Here's the drawing with two shaded views (mm, measured from the low corner). I have some questions. Round coordinates to 2 decimals unless told otherwise and drop trailing zeros. Loops run counter-clockwise (first coordinate to the right, second up) from the corner with the lowest first, then second, coordinate; pieces in that order, holes last.
(1) I want a section at B-B on y = 9. Write out the boundary of the cut face in (x, z).
(2) Will these pins go through, and if not, where does the flat tip stop? pin 1 Ø1.8 at (x, z) = (25, 7.5) entering from -Y; pin 2 Ø1.6 at (x, z) = (31.5, 0.5) entering from -Y; pin 3 Ø10 at (x, y) = (23.5, 45) entering from +Z; pin 4 Ø1.2 at (y, z) = (59, 4) entering from +X.
(3) I want a section at C-C on z = 7.5. Write out the boundary of the cut face in (x, y), plus the area to 3 significant figures.
(4) I want a section at A-A on x = 10. Write out the boundary of the cut face in (y, z).
(5) I want a section at D-D on x = 29. Write out the boundary of the cut face in (y, z).
(6) If I drill on line 1 along X through (y, z) = (51, 0.9); line 2 along Y through (x, z) = (4.5, 0.85); line 3 along Y through (x, z) = (15, 1), over which ranges is the centre line in solid material (lowest first)?
(7) Thinking about a two-plate mould opening in Y: for the marked faces 1, 2, 3 and 4, which applies, released by +Y, released by -Y, zero draft, split by the parting line, or undercut?
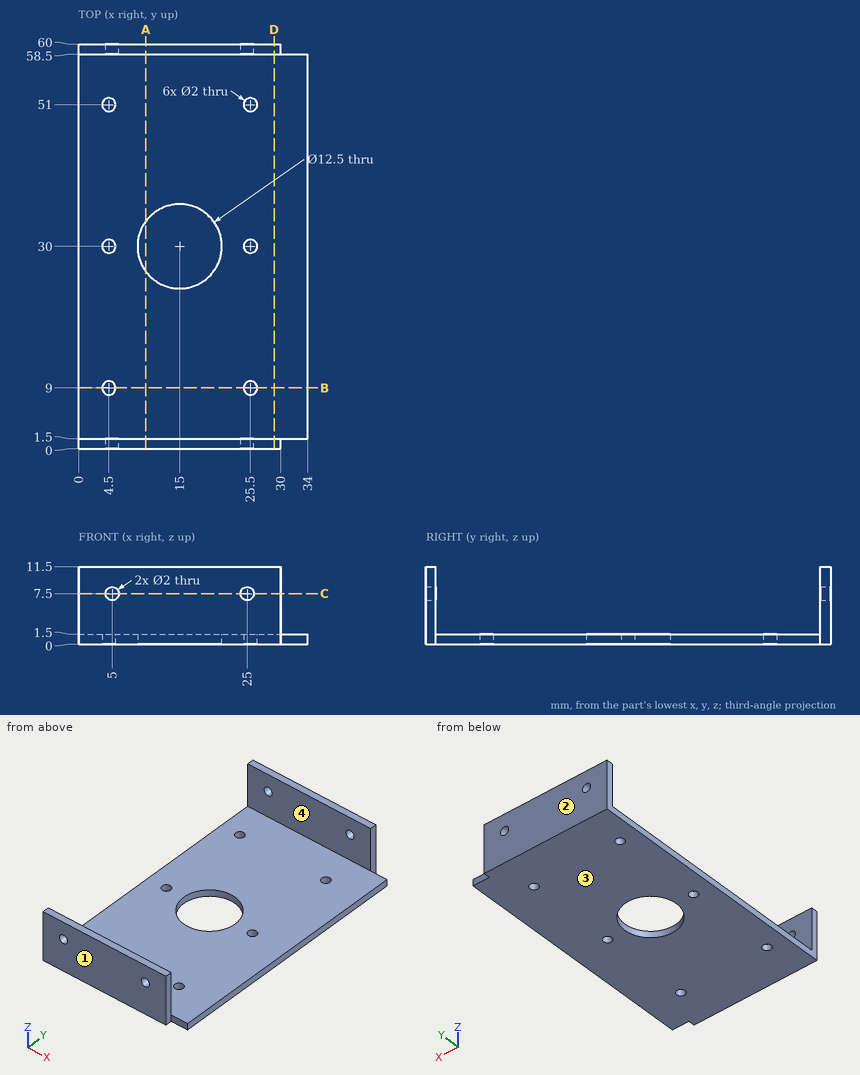
Filled sheet:
1. outline: (0, 0) - (3.5, 0) - (3.5, 1.5) - (0, 1.5) - close; (5.5, 0) - (24.5, 0) - (24.5, 1.5) - (5.5, 1.5) - close; (26.5, 0) - (34, 0) - (34, 1.5) - (26.5, 1.5) - close
2. pin 1: passes through
2. pin 2: stops at y = 1.5
2. pin 3: stops at z = 1.5
2. pin 4: stops at x = 30
3. outline: (0, 0) - (4, 0) - (4, 1.5) - (0, 1.5) - close; (0, 58.5) - (4, 58.5) - (4, 60) - (0, 60) - close; (6, 0) - (24, 0) - (24, 1.5) - (6, 1.5) - close; (6, 58.5) - (24, 58.5) - (24, 60) - (6, 60) - close; (26, 0) - (30, 0) - (30, 1.5) - (26, 1.5) - close; (26, 58.5) - (30, 58.5) - (30, 60) - (26, 60) - close
3. area: 78.0 mm2
4. outline: (0, 0) - (26.25, 0) - (26.25, 1.5) - (1.5, 1.5) - (1.5, 11.5) - (0, 11.5) - close; (33.75, 0) - (60, 0) - (60, 11.5) - (58.5, 11.5) - (58.5, 1.5) - (33.75, 1.5) - close
5. outline: (0, 0) - (60, 0) - (60, 11.5) - (58.5, 11.5) - (58.5, 1.5) - (1.5, 1.5) - (1.5, 11.5) - (0, 11.5) - close
6. line 1: x = 0 to 3.5, 5.5 to 24.5, 26.5 to 34
6. line 2: y = 0 to 8, 10 to 29, 31 to 50, 52 to 60
6. line 3: y = 0 to 23.75, 36.25 to 60
7. face 1: released by -Y
7. face 2: released by +Y
7. face 3: zero draft
7. face 4: undercut
